The listing builds one solid part. Answer for the finished solid, in the listing's coordinates (mm). A direction names the side the tool comes from. Coordinates: 2 decimals unless noted, no trailing zeros. Loops run counter-clockwise (first coordinate to the right, second up) from the corner with the lowest first, then second, coordinate; pieces in that order, holes last. Notation, with made-up numbers: (69, 55) - (83, 55) arc R26 ccw to (83, 78) - close; hole circle Ø11 at (-21, 22.25). An arc over 180 degrees is marked (long way). Write each question's results on one line, items separated by ' | '. Start each with the question number.
(1) Find section D-D on x = 32. Determine the outline of the cut face in (y, z), then the cut area to 3 significant figures.
(2) For faces 1 (the flat face through (-38.4, 0, 1)), 2 (the flat face through (-30, -10, 1)), 3 (the flat face through (39.2, 0, 1)), 4 (the flat face through (35, -10, 1)), determine the directions among +Z, -Z, +X, -X, +Y, -Y from which every point of the face is accessible in a straight line to the end or side of a thin tool.
(3) Consider line 1 (Y direction, x = 0, z = 0.5); line 2 (Y direction, x = -35, z = 0.8); line 3 (X direction, y = -1.5, z = 1.1). Determine where each line is inside the solid, lowest interval first. Write a range as from..to.
(4) Determine the mould class of faces 5 (the cylindrical face through (0, -2, 1)), 6 (the flat face through (-40, -6, 1)), 7 (the flat face through (40, -6, 1)) for opening direction X: released by +X, released by -X, zero draft, split by the parting line, or undercut.
(5) Given pin 1 Ø0.8 at (x, z) = (-39.5, 1) entering from -Y; pin 2 Ø0.8 at (y, z) = (0.5, 0.5) entering from +X, each flat-ended and moving along its own axis, determine where each tip first touches the part or whether it passes through.
(6) Find section B-B on y = 0. Determine the outline of the cut face in (x, z), then the cut area to 3 significant figures.
(7) Find section C-C on z = 1.1. Determine the outline of the cut face in (x, y).
(8) Find section A-A on x = 0. Determine the outline of the cut face in (y, z), then the cut area to 3 significant figures.
from build123d import *

# Parameters (mm, degrees)
CROQUIS1_R              = 2
SALIENTE_EXTRUIR1_DEPTH = 1.5


with BuildPart() as part:
    # Croquis1 → Saliente-Extruir1 (new body)
    with BuildSketch(Plane.XY):
        Polygon((-40, 9.2), (40, 9.2), (40, 1.7), (39.2, 1.7), (39.2, -1.7), (40, -1.7), (40, -10), (30, -10), (30, -10.8), (-30, -10.8), (-30, -9.2), (-40, -9.2), (-40, -2.4), (-38.4, -2.4), (-38.4, 2.4), (-40, 2.4), align=None)
        with Locations((20, 0)):
            Circle(CROQUIS1_R, mode=Mode.SUBTRACT)
        Circle(CROQUIS1_R, mode=Mode.SUBTRACT)
        with Locations((-20, 0)):
            Circle(CROQUIS1_R, mode=Mode.SUBTRACT)
    extrude(amount=SALIENTE_EXTRUIR1_DEPTH)


solid = part.part
Values:
1) outline: (-10, 0) - (9.2, 0) - (9.2, 1.5) - (-10, 1.5) - close | area: 28.8 mm²
2) face 1: +Z, -Z, -X | face 2: +Z, -Z, -X, -Y | face 3: +Z, -Z, +X | face 4: +Z, -Z, +X, -Y
3) line 1: y = -10.8..-2, 2..9.2 | line 2: y = -9.2..9.2 | line 3: x = -38.4..-21.32, -18.68..-1.32, 1.32..18.68, 21.32..39.2
4) face 5: undercut | face 6: released by -X | face 7: released by +X
5) pin 1: stops at y = -9.2 | pin 2: stops at x = 39.2
6) outline: (-38.4, 0) - (-22, 0) - (-22, 1.5) - (-38.4, 1.5) - close; (-18, 0) - (-2, 0) - (-2, 1.5) - (-18, 1.5) - close; (2, 0) - (18, 0) - (18, 1.5) - (2, 1.5) - close; (22, 0) - (39.2, 0) - (39.2, 1.5) - (22, 1.5) - close | area: 98.4 mm²
7) outline: (-40, -9.2) - (-30, -9.2) - (-30, -10.8) - (30, -10.8) - (30, -10) - (40, -10) - (40, -1.7) - (39.2, -1.7) - (39.2, 1.7) - (40, 1.7) - (40, 9.2) - (-40, 9.2) - (-40, 2.4) - (-38.4, 2.4) - (-38.4, -2.4) - (-40, -2.4) - close; hole circle Ø4 at (-20, 0); hole circle Ø4 at (0, 0); hole circle Ø4 at (20, 0)
8) outline: (-10.8, 0) - (-2, 0) - (-2, 1.5) - (-10.8, 1.5) - close; (2, 0) - (9.2, 0) - (9.2, 1.5) - (2, 1.5) - close | area: 24.0 mm²
